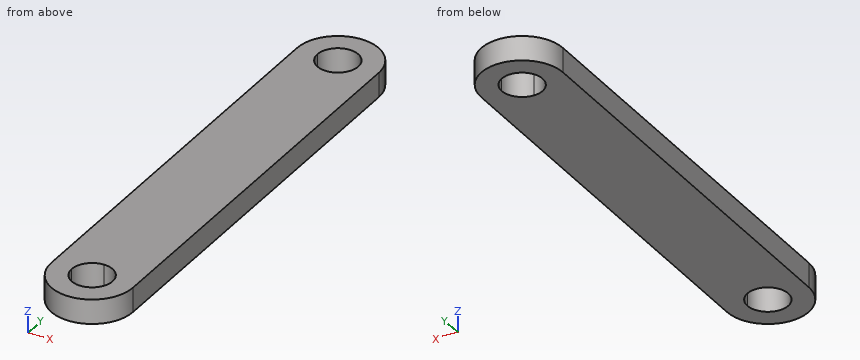
```python
from build123d import *

# Parameters (mm, degrees)
F1_DEPTH = 3.81


with BuildPart() as f1:
    # F0 (on Top) → F1 (new body)
    with BuildSketch(Plane.XY):
        with BuildLine():
            Line((0, 0), (0, 29.21))
            ThreePointArc((0, 29.21), (-2.245064, 30.139936), (-3.175, 32.385))
            Line((-3.175, 32.385), (-6.35, 32.385))
            Line((-6.35, 32.385), (-6.35, -32.385))
            Line((-6.35, -32.385), (-3.175, -32.385))
            ThreePointArc((-3.175, -32.385), (-2.245064, -30.139936), (0, -29.21))
            Line((0, -29.21), (0, 0))
        make_face()
        with BuildLine():
            ThreePointArc((3.175, 32.385), (2.245064, 30.139936), (0, 29.21))
            Line((0, 29.21), (0, 0))
            Line((0, 0), (0, -29.21))
            ThreePointArc((0, -29.21), (2.245064, -30.139936), (3.175, -32.385))
            Line((3.175, -32.385), (6.35, -32.385))
            Line((6.35, -32.385), (6.35, 32.385))
            Line((6.35, 32.385), (3.175, 32.385))
        make_face()
        with BuildLine():
            ThreePointArc((-3.175, 32.385), (0, 35.56), (3.175, 32.385))
            Line((3.175, 32.385), (6.35, 32.385))
            ThreePointArc((6.35, 32.385), (0, 38.735), (-6.35, 32.385))
            Line((-6.35, 32.385), (-3.175, 32.385))
        make_face()
        with BuildLine():
            ThreePointArc((-6.35, -32.385), (0, -38.735), (6.35, -32.385))
            Line((6.35, -32.385), (3.175, -32.385))
            ThreePointArc((3.175, -32.385), (0, -35.56), (-3.175, -32.385))
            Line((-3.175, -32.385), (-6.35, -32.385))
        make_face()
    extrude(amount=F1_DEPTH)


solid = f1.part
```
Check sheet for the modelled part. Datum: model origin and axes. Units: mm. Round coordinates to 2 decimals unless told otherwise and drop trailing zeros. Order: outer loops, then holes, each group sorted by start corner. A loop starts at its lowest first (then second) coordinate and runs counter-clockwise, first axis right, second up. Notation, with made-up numbers: M 24,30.25 L 69,30.25 A12 ccw 69,35.25 Z; hole C 85.25,7 d2. An arc over 180 degrees is marked long. Answer in a Markdown table with one row per item.
(1) Section check D-D on x = -2. Record the boundary of the cut face in (y, z), plus the area to 3 significant figures.
Findings:
| item | result |
|---|---|
| outline | M -38.41,0 L -34.85,0 L -34.85,3.81 L -38.41,3.81 Z; M -29.92,0 L 29.92,0 L 29.92,3.81 L -29.92,3.81 Z; M 34.85,0 L 38.41,0 L 38.41,3.81 L 34.85,3.81 Z |
| area | 255 mm^2 |
(2) Section check C-C on x = 1.25. Record the boundary of the cut face in (y, z).
Findings:
| item | result |
|---|---|
| outline | M -38.61,0 L -35.3,0 L -35.3,3.81 L -38.61,3.81 Z; M -29.47,0 L 29.47,0 L 29.47,3.81 L -29.47,3.81 Z; M 35.3,0 L 38.61,0 L 38.61,3.81 L 35.3,3.81 Z |
(3) Section check A-A on z = 2.2. Record the boundary of the cut face in (x, y) (3 decimals), plus the area to 3 significant figures.
Findings:
| item | result |
|---|---|
| outline | M -6.35,-32.385 A6.35 ccw 6.35,-32.385 L 6.35,32.385 A6.35 ccw -6.35,32.385 Z; hole C 0,-32.385 d6.35; hole C 0,32.385 d6.35 |
| area | 886 mm^2 |
(4) Section check B-B on y = 30. Record the boundary of the cut face in (x, z), plus the area to 3 significant figures.
Findings:
| item | result |
|---|---|
| outline | M -6.35,0 L -2.1,0 L -2.1,3.81 L -6.35,3.81 Z; M 2.1,0 L 6.35,0 L 6.35,3.81 L 2.1,3.81 Z |
| area | 32.4 mm^2 |
(5) Material ranges on line 1 along Y through (x, z) = (0.5, 1.6); line 2 along Y through (x, z) = (-2.25, 0.2); line 3 along X through (y, z) = (33, 3.05), recorded low to high. Write a range as from..to.
Findings:
| item | result |
|---|---|
| line 1 | y = -38.72..-35.52, -29.25..29.25, 35.52..38.72 |
| line 2 | y = -38.32..-34.63, -30.14..30.14, 34.63..38.32 |
| line 3 | x = -6.32..-3.11, 3.11..6.32 |
